```python
from build123d import *

# Parameters (mm, degrees)
SKETCH1_W           = 30.1625
SKETCH1_H           = 38.1
BOSS_EXTRUDE1_DEPTH = 5.0546


with BuildPart() as part:
    # Sketch1 → Revolve1 (revolve)
    with BuildSketch(Plane.XY):
        with Locations((-15.08125, 19.05)):
            Rectangle(SKETCH1_W, SKETCH1_H)
    revolve(axis=Axis((0, 0, 0), (0, -1, 0)))

    # Sketch2 → Boss-Extrude1 (add)
    with BuildSketch(Plane.XZ):
        Polygon((0, 32.647654741), (-23.085378057, 23.085378057), (-32.647654741, 0), (-23.085378057, -23.085378057), (0, -32.647654741), (23.085378057, -23.085378057), (32.647654741, 0), (23.085378057, 23.085378057), align=None)
    extrude(amount=-BOSS_EXTRUDE1_DEPTH)

    # Sketch4 → 3/4 NPT Tapped Hole1 (revolve, cut)
    with BuildSketch(Plane(origin=(0, 0, 0), x_dir=(0, 0, -1), z_dir=(1, 0, 0))):
        Polygon((0, 0), (0, 38.1), (11.5062, 38.1), (11.5062, 14.05382), (12.137858809, 14.05382), (12.558649, 0), align=None)
    revolve(axis=Axis((0, -6.35, 0), (0, 1, 0)), mode=Mode.SUBTRACT)


solid = part.part
```
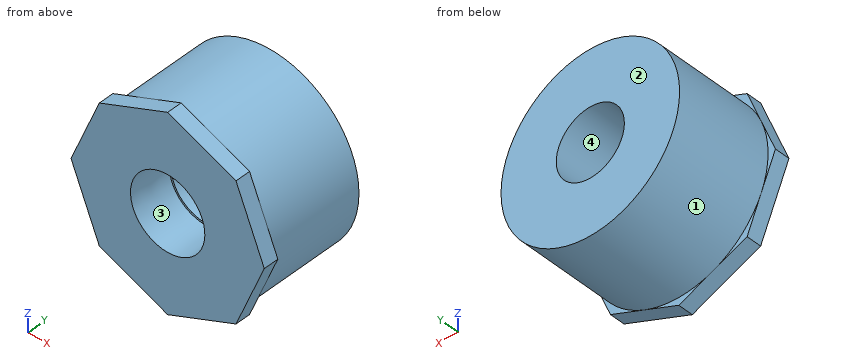
Can you work these out from the model? Positions are in its coordinate system, mm. Face numbers are marked on the shaded views. Give positions to 0.01 mm unless a question says otherwise; leave off trailing zeros. Loops run counter-clockwise (first coordinate to the right, second up) from the corner with the lowest first, then second, coordinate; pieces in that order, holes last. Notation, with made-up numbers: M 64.5,8 L 104.5,8 A11 ccw 104.5,25 Z; hole C 34.5,-5 d5. An arc over 180 degrees is marked long. Use CSV: the item, a comma, the result in double quotes. Start each with the question number.
1. For P1, Ø5, axis at x = -3.5, y = 25, coming from the +Z side; P2, Ø6, axis at y = 13.5, z = 8.5, coming from the -X side; P3, Ø4, axis at x = -22.5, y = 33, coming from the -Z side, each with a flat end and sliding along its axis, tell me the tip position at first contact or that it passes through.
2. Imagine slicing it at C-C, the plane y = 8. Write out the boundary of the cut face in (x, z) (1 decimal).
3. Imagine slicing it at B-B, the plane x = -18.5. Write out the boundary of the cut face in (y, z).
4. If we mould it in two halves opening along Z, with no side actions, what happens to the marked faces 1, 2, 3 and 4? For each: released by +Z, released by -Z, zero draft, split by the parting line, or undercut.
5. Imagine slicing it at A-A, the plane y = 32.5. Write out the boundary of the cut face in (x, z) (1 decimal).
6. If I drill on L1, parallel to Z at x = 0, y = 21.5; L2, parallel to Z at x = 3.5, y = 23.5, over which ranges is the centre line in solid material (lowest first)?
Response values:
1,P1,"z = 30.15"
1,P2,"x = -29.66"
1,P3,"z = -22.13"
2,outline,"C 0,0 d60.3; hole C 0,0 d24.6"
3,outline,"M 0,-24.98 L 5.05,-24.98 L 5.05,-23.82 L 38.1,-23.82 L 38.1,23.82 L 5.05,23.82 L 5.05,24.98 L 0,24.98 Z"
4,face 1,"split by the parting line"
4,face 2,"zero draft"
4,face 3,"undercut"
4,face 4,"undercut"
5,outline,"C 0,0 d60.3; hole C 0,0 d23"
6,L1,"-30.16 to -11.51, 11.51 to 30.16"
6,L2,"-29.96 to -10.96, 10.96 to 29.96"
